Geometry check sheet. Reference: the model listing, model coordinates, mm. Face numbers are marked on the shaded views. A direction names the side the tool comes from. Give positions to 0.01 mm unless a question says otherwise; leave off trailing zeros. Write each loop counter-clockwise with the first axis right and the second up, starting at its lowest first coordinate (ties: lowest second). Pieces come first, ordered by that corner, then holes. Notation, with made-up numbers: (28, 66) - (53, 66) arc R24 cw to (53, 95) - close; hole circle Ø8 at (65, 88). An arc over 180 degrees is marked (long way). One line per question, with ' | ' between items. Start each with the question number.
Q1. Section check C-C on y = 7. Record the boundary of the cut face in (x, z).
Q2. Section check D-D on z = -55. Record the boundary of the cut face in (x, y) (3 decimals).
Q3. Set-up check for the marked faces 1 and 2: record each of +Z, -Z, +X, -X, +Y, -Y from which the full face is reachable in a straight line by a thin tool's end or side.
Q4. Section check B-B on x = 0.5. Record the boundary of the cut face in (y, z) (3 decimals).
Q5. Gauge pin test, flat ends, axial feed: P1, Ø5.5, axis at x = -35.19, y = 0, coming from the -Z side; P2, Ø10, axis at y = 3.5, z = 37.5, coming from the -X side. Record the tip position at first contact, or that the pin passes through.
Q6. Thickness scan on L1, parallel to X at y = 0, z = 81; L2, parallel to Z at x = 37, y = -3.75; L3, parallel to X at y = 8.75, z = 48. Record the ranges inside material, lowest first. Write a range as [from, to].
Q7. Section check A-A on y = 0. Count the separate pieces of the cut face and the enclosed holes in it, and give its area (3 significant figures).
```python
from build123d import *

# Parameters (mm, degrees)
SKETCH3_W                       = 89.4306822
SKETCH3_H                       = 19.05
BOSS_EXTRUDE1_DEPTH             = 82.538333314
SKETCH4_W                       = 87.5256822
SKETCH4_H                       = 161.266666628
CUT_EXTRUDE1_DEPTH              = 96.785910738
F_6_CLEARANCE_HOLE1_AT_2_COUNT  = 2
F_6_CLEARANCE_HOLE1_AT_2_PITCH  = 70.3806822
F_6_CLEARANCE_HOLE2_D           = 4.3053
F_6_CLEARANCE_HOLE2_DEPTH       = 6.858
F_6_CLEARANCE_HOLE2_CSINK_D     = 6.6548
F_6_CLEARANCE_HOLE2_CSINK_ANGLE = 90
F_6_CLEARANCE_HOLE2_TIP         = 1.293442612


with BuildPart() as part:
    # Sketch3 → Boss-Extrude1 (new, symmetric)
    with BuildSketch(Plane.XY):
        Rectangle(SKETCH3_W, SKETCH3_H)
    extrude(amount=BOSS_EXTRUDE1_DEPTH, both=True)

    # Sketch4 → Cut-Extrude1 (cut, through all)
    with BuildSketch(Plane.XZ.offset(9.525)):
        with Locations((-0.9525, 0)):
            Rectangle(SKETCH4_W, SKETCH4_H)
    extrude(amount=-CUT_EXTRUDE1_DEPTH, mode=Mode.SUBTRACT)

    # Sketch6 → #6 Clearance Hole1 (revolve, cut)
    with BuildSketch(Plane(origin=(35.1903411, 0, -82.538333314), x_dir=(0, 1, 0), z_dir=(1, 0, 0))):
        Polygon((0, 0), (0, 1.905), (2.15265, 1.905), (2.15265, 1.17475), (3.3274, 0), align=None)
    f_6_clearance_hole1 = revolve(axis=Axis((35.1903411, 0, -88.888333314), (0, 0, 1)), mode=Mode.SUBTRACT)

    # #6 Clearance Hole1 at 2: #6 Clearance Hole1 ×2
    with Locations(*[(-i * F_6_CLEARANCE_HOLE1_AT_2_PITCH, 0, 0) for i in range(1, F_6_CLEARANCE_HOLE1_AT_2_COUNT)]):
        add(f_6_clearance_hole1, mode=Mode.SUBTRACT)

    # #6 Clearance Hole2
    with Locations(Plane.XY.offset(82.538333314)):
        with Locations((-35.1903411, 0), (35.1903411, 0)):
            CounterSinkHole(F_6_CLEARANCE_HOLE2_D / 2, F_6_CLEARANCE_HOLE2_CSINK_D / 2, depth=F_6_CLEARANCE_HOLE2_DEPTH, counter_sink_angle=F_6_CLEARANCE_HOLE2_CSINK_ANGLE)
            with Locations((0, 0, -(F_6_CLEARANCE_HOLE2_DEPTH + F_6_CLEARANCE_HOLE2_TIP / 2))):  # 118° drill point
                Cone(0, F_6_CLEARANCE_HOLE2_D / 2, F_6_CLEARANCE_HOLE2_TIP, mode=Mode.SUBTRACT)


solid = part.part
```
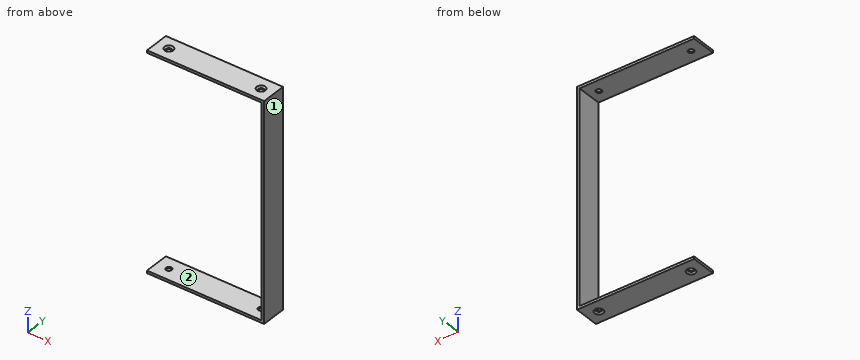
Working result:
1) outline: (-44.72, -82.54) - (44.72, -82.54) - (44.72, 82.54) - (-44.72, 82.54) - (-44.72, 80.63) - (42.81, 80.63) - (42.81, -80.63) - (-44.72, -80.63) - close
2) outline: (42.81, -9.525) - (44.715, -9.525) - (44.715, 9.525) - (42.81, 9.525) - close
3) face 1: +Z, -Z, +X, +Y, -Y | face 2: -X, +Y, -Y
4) outline: (-9.525, -82.538) - (9.525, -82.538) - (9.525, -80.633) - (-9.525, -80.633) - close; (-9.525, 80.633) - (9.525, 80.633) - (9.525, 82.538) - (-9.525, 82.538) - close
5) P1: stops at z = -81.96 | P2: stops at x = 42.81
6) L1: x = [-44.72, -37.34], [-33.04, 33.04], [37.34, 44.72] | L2: z = [-82.54, -80.63], [80.63, 82.54] | L3: x = [42.81, 44.72]
7) separate pieces: 5 | enclosed holes: 0 | area: 610 mm2
